```python
from build123d import *

# Parameters (mm, degrees)
SKETCH_1_W          = 368
SKETCH_1_H          = 368
EXTRUDE_1_DEPTH     = 4
SKETCH_3_R          = 2.55
CUT_EXTRUDE_2_DEPTH = 261.246037434
SKETCH_4_W          = 20
SKETCH_4_H          = 20
CUT_EXTRUDE_3_DEPTH = 261.246037434
SKETCH_5_R          = 2.5
CUT_EXTRUDE_6_DEPTH = 10
SKETCH_6_R          = 2
SKETCH_6_R_2        = 2.0450624
SKETCH_6_R_3        = 2.5
CUT_EXTRUDE_7_DEPTH = 10


with BuildPart() as part:
    # 草图1 → 凸台-拉伸1 (new body)
    with BuildSketch(Plane.XY):
        Rectangle(SKETCH_1_W, SKETCH_1_H)
    extrude(amount=EXTRUDE_1_DEPTH)

    # 草图3 → 切除-拉伸2 (cut, through all)
    with BuildSketch(Plane.XY.offset(4)):
        with Locations((0, -175)):
            Circle(SKETCH_3_R)
        with Locations((70, -175)):
            Circle(SKETCH_3_R)
        with Locations((140, -175)):
            Circle(SKETCH_3_R)
        with Locations((-70, -175)):
            Circle(SKETCH_3_R)
        with Locations((-140, -175)):
            Circle(SKETCH_3_R)
        with Locations((-175, 140)):
            Circle(SKETCH_3_R)
        with Locations((-175, 70)):
            Circle(SKETCH_3_R)
        with Locations((-175, -70)):
            Circle(SKETCH_3_R)
        with Locations((-175, -140)):
            Circle(SKETCH_3_R)
        with Locations((-175, 0)):
            Circle(SKETCH_3_R)
        with Locations((140, 175)):
            Circle(SKETCH_3_R)
        with Locations((70, 175)):
            Circle(SKETCH_3_R)
        with Locations((-70, 175)):
            Circle(SKETCH_3_R)
        with Locations((-140, 175)):
            Circle(SKETCH_3_R)
        with Locations((0, 175)):
            Circle(SKETCH_3_R)
        with Locations((175, -140)):
            Circle(SKETCH_3_R)
        with Locations((175, -70)):
            Circle(SKETCH_3_R)
        with Locations((175, 70)):
            Circle(SKETCH_3_R)
        with Locations((175, 140)):
            Circle(SKETCH_3_R)
        with Locations((175, 0)):
            Circle(SKETCH_3_R)
    extrude(amount=-CUT_EXTRUDE_2_DEPTH, mode=Mode.SUBTRACT)

    # 草图4 → 切除-拉伸3 (cut, through all)
    with BuildSketch(Plane.XY.offset(4)):
        with Locations((-174, 174)):
            Rectangle(SKETCH_4_W, SKETCH_4_H)
        with Locations((-174, -174)):
            Rectangle(SKETCH_4_W, SKETCH_4_H)
        with Locations((174, 174)):
            Rectangle(SKETCH_4_W, SKETCH_4_H)
        with Locations((174, -174)):
            Rectangle(SKETCH_4_W, SKETCH_4_H)
    extrude(amount=-CUT_EXTRUDE_3_DEPTH, mode=Mode.SUBTRACT)

    # 草图5 → 切除-拉伸6 (cut)
    with BuildSketch(Plane.XY.offset(4)):
        Circle(SKETCH_5_R)
        with Locations((-15.909902577, 15.909902577)):
            Circle(SKETCH_5_R)
        with Locations((15.909902577, 15.909902577)):
            Circle(SKETCH_5_R)
        with Locations((15.909902577, -15.909902577)):
            Circle(SKETCH_5_R)
        with Locations((-15.909902577, -15.909902577)):
            Circle(SKETCH_5_R)
    extrude(amount=-CUT_EXTRUDE_6_DEPTH, mode=Mode.SUBTRACT)

    # 草图6 → 切除-拉伸7 (cut)
    with BuildSketch(Plane(origin=(0, 0, 0), x_dir=(-1, 0, 0), z_dir=(0, 0, -1))):
        with Locations((121.8, -122)):
            Circle(SKETCH_6_R)
        with Locations((71.8, -72)):
            Circle(SKETCH_6_R)
        with Locations((-72, -122)):
            Circle(SKETCH_6_R)
        with Locations((-122, -72)):
            Circle(SKETCH_6_R)
        with Locations((-72, 64)):
            Circle(SKETCH_6_R)
        with Locations((-122, 114)):
            Circle(SKETCH_6_R)
        with Locations((121.8, 64)):
            Circle(SKETCH_6_R_2)
        with Locations((71.8, 114)):
            Circle(SKETCH_6_R)
        with Locations((105.553117778, -14)):
            Circle(SKETCH_6_R_3)
        with Locations((105.553117778, 2)):
            Circle(SKETCH_6_R_3)
        with Locations((54.253117778, -14)):
            Circle(SKETCH_6_R_3)
        with Locations((54.253117778, 2)):
            Circle(SKETCH_6_R_3)
    extrude(amount=-CUT_EXTRUDE_7_DEPTH, mode=Mode.SUBTRACT)


solid = part.part
```
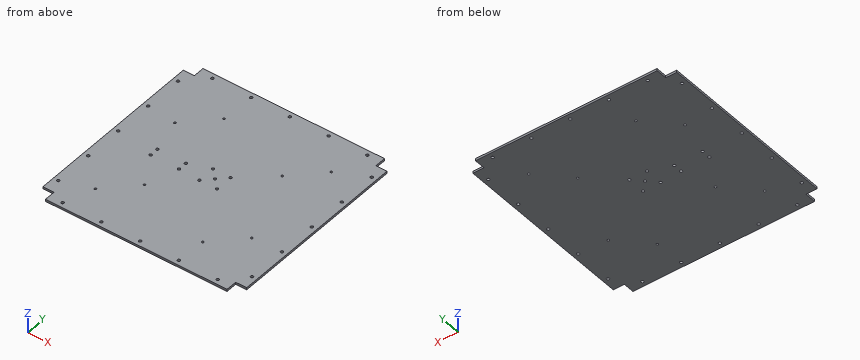
Input: part model. Units: mm. Frame: model coordinates. Coordinates: 2 decimals unless noted, no trailing zeros. Use a Markdown table: item, result. Add a question column.
1) Section A-A, the plane z = 3.1. Give the number of separate pieces and of enclosed holes in the cut face, plus the area to 3 significant figures.
2) Line query: L1, parallel to X at y = 175, z = 0.95; L2, parallel to X at y = -122.5, z = 1.35; L3, parallel to Y at x = 140, z = 1.55. Output: solid intervals per line, ascending. Write a range as from..to.
3) Pin query (flat end, axial travel): P1, Ø6, axis at x = 140, y = 175, coming from the +Z side; P2, Ø1.2, axis at y = -174.5, z = 1.5, coming from the -X side. Return the tip coordinate at first contact, or that it passes through.
Answer below:
| question | item | result |
|---|---|---|
| 1 | separate pieces | 1 |
| 1 | enclosed holes | 37 |
| 1 | area | 133,000 mm2 |
| 2 | L1 | -164..-142.55, -137.45..-72.55, -67.45..-2.55, 2.55..67.45, 72.55..137.45, 142.55..164 |
| 2 | L2 | -184..-123.74, -119.86..70.06, 73.94..184 |
| 2 | L3 | -184..-177.55, -172.45..172.45, 177.55..184 |
| 3 | P1 | z = 4 |
| 3 | P2 | x = -164 |
